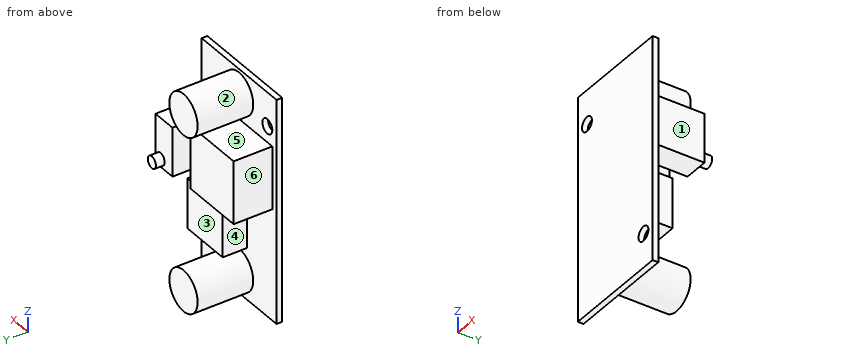
from build123d import *

# Parameters (mm, degrees)
SKETCH_1_W      = 21.2
SKETCH_1_H      = 43.5
SKETCH_1_R      = 1.4
EXTRUDE_1_DEPTH = 1.1
SKETCH_2_R      = 4
EXTRUDE_2_DEPTH = 10.8
SKETCH_3_W      = 12.2
SKETCH_3_H      = 12.2
EXTRUDE_3_DEPTH = 7.5
SKETCH_4_W      = 4.8
SKETCH_4_H      = 9.5
EXTRUDE_4_DEPTH = 10.2
SKETCH_5_W      = 10
SKETCH_5_H      = 9.7
EXTRUDE_5_DEPTH = 4.7
SKETCH_6_R      = 1.15
EXTRUDE_6_DEPTH = 1.7


with BuildPart() as part:
    # 草图1 → 凸台-拉伸1 (new body)
    with BuildSketch(Plane(origin=(0, 0, 0), x_dir=(1, 0, 0), z_dir=(0, 1, 0))):
        Rectangle(SKETCH_1_W, SKETCH_1_H)
        with Locations((8, 15.15)):
            Circle(SKETCH_1_R, mode=Mode.SUBTRACT)
        with Locations((-8, -15.15)):
            Circle(SKETCH_1_R, mode=Mode.SUBTRACT)
    extrude(amount=EXTRUDE_1_DEPTH)

    # 草图2 → 凸台-拉伸2 (add)
    with BuildSketch(Plane(origin=(0, 1.1, 0), x_dir=(1, 0, 0), z_dir=(0, 1, 0))):
        with Locations((0, 17.1)):
            Circle(SKETCH_2_R)
        with Locations((0, -17.1)):
            Circle(SKETCH_2_R)
    extrude(amount=EXTRUDE_2_DEPTH)

    # 草图3 → 凸台-拉伸3 (add)
    with BuildSketch(Plane(origin=(0, 1.1, 0), x_dir=(1, 0, 0), z_dir=(0, 1, 0))):
        with Locations((-3.3, -5.95)):
            Rectangle(SKETCH_3_W, SKETCH_3_H)
    extrude(amount=EXTRUDE_3_DEPTH)

    # 草图4 → 凸台-拉伸4 (add)
    with BuildSketch(Plane(origin=(0, 1.1, 0), x_dir=(1, 0, 0), z_dir=(0, 1, 0))):
        with Locations((6.4, -7.3)):
            Rectangle(SKETCH_4_W, SKETCH_4_H)
    extrude(amount=EXTRUDE_4_DEPTH)

    # 草图5 → 凸台-拉伸5 (add)
    with BuildSketch(Plane(origin=(0, 1.1, 0), x_dir=(1, 0, 0), z_dir=(0, 1, 0))):
        with Locations((2.8, 6.9)):
            Rectangle(SKETCH_5_W, SKETCH_5_H)
    extrude(amount=EXTRUDE_5_DEPTH)

    # 草图6 → 凸台-拉伸6 (add)
    with BuildSketch(Plane(origin=(0, 11.3, 0), x_dir=(1, 0, 0), z_dir=(0, 1, 0))):
        with Locations((7.351662329, -4.096039532)):
            Circle(SKETCH_6_R)
    extrude(amount=EXTRUDE_6_DEPTH)


solid = part.part
Source: CAD feature listing. Evaluate the final solid. Frame: model axes, mm. Face numbers are marked on the shaded views. A direction names the side the tool comes from. Coordinates: 2 decimals unless noted, no trailing zeros. Loops run counter-clockwise (first coordinate to the right, second up) from the corner with the lowest first, then second, coordinate; pieces in that order, holes last. Notation, with made-up numbers: (-19.75, 40) -> (20.25, 40) arc R14 cw to (20.25, 51) -> close; hole circle Ø3 at (60, -24). An arc over 180 degrees is marked (long way). Answer in a Markdown table with one row per item. Add a question column.
Q1. Ray query, line 1 along Z through (x, y) = (8, 0.75); line 2 along Z through (x, y) = (0, 6.25); line 3 along X through (y, z) = (0.35, 15.15). Return the intervals inside material, ascending.
Q2. Reachability of the marked faces 1, 2, 3 and 4 from +Z, -Z, +X, -X, +Y, -Y: full face, straight path, thin tool, end or side. Return the list, or none.
Q3. Section D-D on x = 0. Return the cut outline in (y, z), and give its area (3 significant figures).
Q4. Pull-direction query (Z, two-part tool) for the marked faces 5 and 6; classes: pulls with the +Z half, pulls with the -Z half, needs draft (parallel to the pull), parting line crosses it, or undercut.
Q5. Section A-A on x = -8. Return the cut outline in (y, z).
Q6. Section C-C on z = -15.15. Return the cut outline in (x, y).
Q7. Contact query for flat-ended pins moving along their axis: pin 1 Ø2 at (x, z) = (2.5, -16) entering from +Y; pin 2 Ø6 at (y, z) = (6.5, 8.5) entering from -X; pin 3 Ø4 at (y, z) = (5, 5) entering from +X. Output: stop coordinate, or through.
Q8. Section B-B on z = -9.5. Return the cut outline in (x, y), and give its area (3 significant figures).
Computed values:
| question | item | result |
|---|---|---|
| 1 | line 1 | z = -21.75 to -16.55, -13.75 to 21.75 |
| 1 | line 2 | z = -21.1 to -13.1, -0.15 to 12.05, 13.1 to 21.1 |
| 1 | line 3 | x = -10.6 to -9.4, -6.6 to 10.6 |
| 2 | face 1 | +Z, -Z, +X, +Y |
| 2 | face 2 | +Y |
| 2 | face 3 | +X, -X, +Y |
| 2 | face 4 | -X, +Y |
| 3 | outline | (0, -21.75) -> (1.1, -21.75) -> (1.1, -21.1) -> (11.9, -21.1) -> (11.9, -13.1) -> (1.1, -13.1) -> (1.1, -11.75) -> (5.8, -11.75) -> (5.8, -2.05) -> (1.1, -2.05) -> (1.1, -0.15) -> (8.6, -0.15) -> (8.6, 12.05) -> (1.1, 12.05) -> (1.1, 13.1) -> (11.9, 13.1) -> (11.9, 21.1) -> (1.1, 21.1) -> (1.1, 21.75) -> (0, 21.75) -> close |
| 3 | area | 358 mm^2 |
| 4 | face 5 | undercut |
| 4 | face 6 | needs draft |
| 5 | outline | (0, -21.75) -> (1.1, -21.75) -> (1.1, -0.15) -> (8.6, -0.15) -> (8.6, 12.05) -> (1.1, 12.05) -> (1.1, 13.75) -> (0, 13.75) -> close; (0, 16.55) -> (1.1, 16.55) -> (1.1, 21.75) -> (0, 21.75) -> close |
| 6 | outline | (-10.6, 0) -> (6.6, 0) -> (6.6, 1.1) -> (3.49, 1.1) -> (3.49, 11.9) -> (-3.49, 11.9) -> (-3.49, 1.1) -> (-10.6, 1.1) -> close; (9.4, 0) -> (10.6, 0) -> (10.6, 1.1) -> (9.4, 1.1) -> close |
| 7 | pin 1 | stops at y = 11.9 |
| 7 | pin 2 | stops at x = -9.4 |
| 7 | pin 3 | stops at x = 8.8 |
| 8 | outline | (-10.6, 0) -> (10.6, 0) -> (10.6, 1.1) -> (7.8, 1.1) -> (7.8, 5.8) -> (-2.2, 5.8) -> (-2.2, 1.1) -> (-10.6, 1.1) -> close |
| 8 | area | 70.3 mm^2 |
